Input: part model. Units: mm. Frame: model coordinates. A direction names the side the tool comes from. Coordinates: 2 decimals unless noted, no trailing zeros. Loops run counter-clockwise (first coordinate to the right, second up) from the corner with the lowest first, then second, coordinate; pieces in that order, holes last.
Item 1: Contact query for a flat-ended pin moving along its axis: P1, Ø1.5, axis at x = 17.5, y = 24.5, coming from the -Z side. Output: stop coordinate, or through.
Item 2: Ray query, line 1 along Y through (x, z) = (11.75, 24.5); line 2 along X through (y, z) = (28.5, -98.5). Return the intervals inside material, ascending.
Item 3: Pull-direction query (Y, two-part tool) for faces 3 (the flat face through (10, 0, 3)), 4 (the flat face through (10, 1.5, 3)), 5 (the flat face through (1, 22, 215)); classes: released by +Y, released by -Y, zero draft, split by the parting line, or undercut.
Item 4: Section A-A on x = 10.75. Return loops of the section in (y, z), and give its area (3 significant figures).
Item 5: Section B-B on y = 15. Return loops of the section in (x, z).
Item 6: Reachability of faces 1 (the flat face through (1, 22, -215)), 2 (the flat face through (1.5, 20, 3)) from +Z, -Z, +X, -X, +Y, -Y: full face, straight path, thin tool, end or side. Return the list, or none.
Item 7: Section C-C on z = -7.5. Return loops of the section in (x, y), and give its area (3 significant figures).
```python
from build123d import *

# Parameters (mm, degrees)
EXTRUDE_1_DEPTH = 215


# Read off the part's stored shape, not the designer's step: Бобышка-Вытянуть1
with BuildPart() as part:
    # Бобышка-Вытянуть1 outline → Бобышка-Вытянуть1 (new body)
    with BuildSketch(Plane.XY):
        with BuildLine():
            ThreePointArc((20, 38.5), (19.560660172, 39.560660172), (18.5, 40))
            Line((18.5, 40), (1.5, 40))
            ThreePointArc((1.5, 40), (0.439339828, 39.560660172), (0, 38.5))
            Line((0, 38.5), (0, 1.5))
            ThreePointArc((0, 1.5), (0.439339828, 0.439339828), (1.5, 0))
            Line((1.5, 0), (18.5, 0))
            ThreePointArc((18.5, 0), (19.560660172, 0.439339828), (20, 1.5))
            Line((20, 1.5), (20, 38.5))
        make_face()
        with BuildLine():
            Line((18.5, 37.5), (18.5, 2.5))
            ThreePointArc((18.5, 2.5), (18.207106781, 1.792893219), (17.5, 1.5))
            Line((17.5, 1.5), (2.5, 1.5))
            ThreePointArc((2.5, 1.5), (1.792893219, 1.792893219), (1.5, 2.5))
            Line((1.5, 2.5), (1.5, 37.5))
            ThreePointArc((1.5, 37.5), (1.792893219, 38.207106781), (2.5, 38.5))
            Line((2.5, 38.5), (17.5, 38.5))
            ThreePointArc((17.5, 38.5), (18.207106781, 38.207106781), (18.5, 37.5))
        make_face(mode=Mode.SUBTRACT)
    extrude(amount=EXTRUDE_1_DEPTH)

    # Зеркальное отражение2: part across plane


with BuildPart() as part_1:
    add(part.part)
    add(part.part.mirror(Plane(origin=(18.5, 38.5, 0), x_dir=(1, 0, 0), z_dir=(0, 0, -1))))


solid = part_1.part
```
Results found:
1. P1: passes through
2. line 1: y = 0 to 1.5, 38.5 to 40
2. line 2: x = 0 to 1.5, 18.5 to 20
3. face 3: released by -Y
3. face 4: undercut
3. face 5: zero draft
4. outline: (0, -215) - (1.5, -215) - (1.5, 215) - (0, 215) - close; (38.5, -215) - (40, -215) - (40, 215) - (38.5, 215) - close
4. area: 1,290 mm2
5. outline: (0, -215) - (1.5, -215) - (1.5, 215) - (0, 215) - close; (18.5, -215) - (20, -215) - (20, 215) - (18.5, 215) - close
6. face 1: -Z, +X, -X, +Y, -Y
6. face 2: +Z, -Z
7. outline: (0, 1.5) arc R1.5 ccw to (1.5, 0) - (18.5, 0) arc R1.5 ccw to (20, 1.5) - (20, 38.5) arc R1.5 ccw to (18.5, 40) - (1.5, 40) arc R1.5 ccw to (0, 38.5) - close; hole (1.5, 2.5) arc R1 ccw to (2.5, 1.5) - (17.5, 1.5) arc R1 ccw to (18.5, 2.5) - (18.5, 37.5) arc R1 ccw to (17.5, 38.5) - (2.5, 38.5) arc R1 ccw to (1.5, 37.5) - close
7. area: 170 mm2
